```python
from build123d import *

# Parameters (mm, degrees)
SKETCH1_W            = 203.2
SKETCH1_H            = 177.8
SKETCH1_W_2          = 80.17565134
SKETCH1_H_2          = 54.163037222
BOSS_EXTRUDE1_DEPTH  = 2.54
LPATTERN2_COUNT      = 9
LPATTERN2_PITCH      = 20
LPATTERN2_COUNT_DIR2 = 10
LPATTERN2_PITCH_DIR2 = 20


with BuildPart() as part:
    # Sketch1 → Boss-Extrude1 (new body)
    with BuildSketch(Plane.XY):
        Rectangle(SKETCH1_W, SKETCH1_H)
        with Locations((0, -3.553866914)):
            Rectangle(SKETCH1_W_2, SKETCH1_H_2, mode=Mode.SUBTRACT)
    extrude(amount=BOSS_EXTRUDE1_DEPTH)

    # Sketch4 → M2.5 Clearance Hole1 (revolve, cut)
    with BuildSketch(Plane(origin=(91.6, 78.994, 0), x_dir=(0, 1, 0), z_dir=(1, 0, 0))):
        Polygon((0, 0), (0, 5.623506083), (1.75, 4.572), (1.75, 0), align=None)
    m2_5_clearance_hole1 = revolve(axis=Axis((91.6, 78.994, -6.35), (0, 0, 1)), mode=Mode.SUBTRACT)

    # LPattern2: M2.5 Clearance Hole1 9 × 10, 12 skipped
    with Locations(*[(-j * LPATTERN2_PITCH_DIR2, -i * LPATTERN2_PITCH, 0) for i in range(LPATTERN2_COUNT) for j in range(LPATTERN2_COUNT_DIR2) if (i, j) not in ((0, 0), (3, 3), (3, 4), (3, 5), (3, 6), (4, 3), (4, 4), (4, 5), (4, 6), (5, 3), (5, 4), (5, 5), (5, 6))]):
        add(m2_5_clearance_hole1, mode=Mode.SUBTRACT)


solid = part.part
```
CAD build for the part. Positions are in the model's coordinates, mm. Round coordinates to 2 decimals unless told otherwise and drop trailing zeros. Write each loop counter-clockwise with the first axis right and the second up, starting at its lowest first coordinate (ties: lowest second). Pieces come first, ordered by that corner, then holes.
Item 1: Band-saw the part on A-A on x = 23.5. Write the cut outline in (y, z).
Filled in:
outline: (-88.9, 0) - (-30.64, 0) - (-30.64, 2.54) - (-88.9, 2.54) - close; (23.53, 0) - (88.9, 0) - (88.9, 2.54) - (23.53, 2.54) - close
Item 2: Drill centre lines: L1, parallel to Y at x = 4.5, z = 0.45; L2, parallel to X at y = 7.5, z = 0.7. Where is each one in solid material? Low to high.
Filled in:
L1: y = -88.9 to -30.64, 23.53 to 88.9
L2: x = -101.6 to -40.09, 40.09 to 101.6
Item 3: Band-saw the part on B-B on z = 2. Give the number of separate pieces and of enclosed holes in the cut face, then the cut area to 3 significant figures.
Filled in:
separate pieces: 1
enclosed holes: 79
area: 31,000 mm2
Item 4: Drop a flat-ended pin along its axis: pin 1 Ø2 at (x, y) = (-88.4, -1.006) entering from -Z. Give the stop position or say it passes through.
Filled in:
pin 1: passes through
